```python
from build123d import *

# Parameters (mm, degrees)
F0_R         = 23.8211318964
F0_R_2       = 22.0256608
F3_DEPTH     = 50.17713
F3_FACE_R    = 23.8211318964
F3_FACE_R_2  = 22.0256608
F3_FACE1_R   = 23.8211318964
F3_FACE1_R_2 = 22.0256608
F4_DEPTH     = 2.16738
F1_R         = 2.1104987
F5_DEPTH     = 100.6018
F2_W         = 22.9499428533
F2_H         = 0.7366
F2_W_2       = 0.7306225889
F2_H_2       = 22.9688390891
F2_W_3       = 22.9015578225
F2_H_3       = 22.9767380224
F6_DEPTH     = 36.93024


with BuildPart() as f3:
    # F0 (on Top) → F3 (new body)
    with BuildSketch(Plane.XY):
        Circle(F0_R)
        Circle(F0_R_2, mode=Mode.SUBTRACT)
    extrude(amount=F3_DEPTH)

    # F0 (on Top) + F3_face (on face) + F3_face1 (on face) → F4 (join)
    with BuildSketch(Plane.XY):
        Circle(F0_R)
        Circle(F0_R_2, mode=Mode.SUBTRACT)
        Circle(F0_R_2)
    with BuildSketch(Plane.XY.offset(50.17713)):
        Circle(F3_FACE_R)
        Circle(F3_FACE_R_2, mode=Mode.SUBTRACT)
    with BuildSketch(Plane(origin=(0, 0, 0), x_dir=(1, 0, 0), z_dir=(0, 0, -1))):
        Circle(F3_FACE1_R)
        Circle(F3_FACE1_R_2, mode=Mode.SUBTRACT)
    extrude(amount=F4_DEPTH, dir=(0, 0, 1))

    # F1 (on Top) → F5 (join)
    with BuildSketch(Plane.XY):
        Circle(F1_R)
    extrude(amount=F5_DEPTH)

    # F2 (on Top) → F6 (join)
    with BuildSketch(Plane.XY):
        with Locations((11.8395101745, 0.0209339964)):
            Rectangle(F2_W, F2_H)
        with Locations((-0.0007725466, 0.0209339964)):
            Rectangle(F2_W_2, F2_H)
        with Locations((-0.0007725466, 11.873653541)):
            Rectangle(F2_W_2, F2_H_2)
        with Locations((-11.8168627523, 0.0209339964)):
            Rectangle(F2_W_3, F2_H)
        with Locations((-0.0007725466, -11.8357350148)):
            Rectangle(F2_W_2, F2_H_3)
    extrude(amount=F6_DEPTH)


solid = f3.part
```
Verification items for the finished model (mm, model axes). A direction names the side the tool comes from. Coordinates: 2 decimals unless noted, no trailing zeros. Loops run counter-clockwise (first coordinate to the right, second up) from the corner with the lowest first, then second, coordinate; pieces in that order, holes last. Notation, with made-up numbers: (12.25, -34.75) -> (22.25, -34.75) arc R16 ccw to (22.25, -8.75) -> close; hole circle Ø8 at (64, -37.75). An arc over 180 degrees is marked (long way). Answer in a Markdown table with one row per item.
1) Draft check along X on faces 1 (the face through (0.365, 12, 19)), 2 (the face through (-5.164, -23.255, 25.806)), 3 (the face through (0, 0, 0)). Enter one of: released by +X, released by -X, zero draft, split by the parting line, or undercut.
The answers:
| item | result |
|---|---|
| face 1 | undercut |
| face 2 | split by the parting line |
| face 3 | zero draft |
2) Section check D-D (z = 75.5). Record the cut outline in (x, y).
The answers:
| item | result |
|---|---|
| outline | circle Ø4.22 at (0, 0) |
3) Section check A-A (z = 9.5). Record the cut outline in (x, y), and give its area (3 significant figures).
The answers:
| item | result |
|---|---|
| outline | circle Ø47.64 at (0, 0); hole (-22.02, -0.35) arc R22.03 ccw to (-0.37, -22.02) -> (-0.37, -2.08) arc R2.11 cw to (-2.08, -0.35) -> close; hole (-22.02, 0.39) -> (-2.07, 0.39) arc R2.11 cw to (-0.37, 2.08) -> (-0.37, 22.02) arc R22.03 ccw to start; hole (0.36, -22.02) arc R22.03 ccw to (22.02, -0.35) -> (2.08, -0.35) arc R2.11 cw to (0.36, -2.08) -> close; hole (0.36, 2.08) arc R2.11 cw to (2.07, 0.39) -> (22.02, 0.39) arc R22.03 ccw to (0.36, 22.02) -> close |
| area | 331 mm2 |
4) Section check C-C (y = 19). Record the cut outline in (x, z), and give its area (3 significant figures).
The answers:
| item | result |
|---|---|
| outline | (-14.37, 0) -> (14.37, 0) -> (14.37, 52.34) -> (11.14, 52.34) -> (11.14, 2.17) -> (0.36, 2.17) -> (0.36, 36.93) -> (-0.37, 36.93) -> (-0.37, 2.17) -> (-11.14, 2.17) -> (-11.14, 52.34) -> (-14.37, 52.34) -> close |
| area | 412 mm2 |
5) Access from +Z, -Z, +X, -X, +Y, -Y to the whole of each face (thin tool, end or side, straight path). Record for faces 4 (the face through (0, 0, 100.602)), 5 (the face through (-9, -9, 2.167)).
The answers:
| item | result |
|---|---|
| face 4 | +Z, +X, -X, +Y, -Y |
| face 5 | +Z |
6) Depth check by flat-ended pin: P1, Ø6, axis at x = -7.5, z = 25, coming from the +Y side; P2, Ø12, axis at x = 11.5, z = 50, coming from the +Y side; P3, Ø1, axis at x = 9, z = 29, coming from the -Y side; P4, Ø6, axis at x = -6, z = 64, coming from the +Y side. Enter the tip coordinate at first touch or a pass-through.
The answers:
| item | result |
|---|---|
| P1 | stops at y = 23.39 |
| P2 | stops at y = 23.18 |
| P3 | stops at y = -22.25 |
| P4 | passes through |
7) Scan lines: line 1 along X through (y, z) = (0.5, 36); line 2 along X through (y, z) = (-10.5, 16.5); line 3 along Y through (x, z) = (13, 9.5). Record each from-to range of solid material in increasing order. Write a range as from..to.
The answers:
| item | result |
|---|---|
| line 1 | x = -23.82..-22.02, -2.05..2.05, 22.02..23.82 |
| line 2 | x = -21.38..-19.36, -0.37..0.36, 19.36..21.38 |
| line 3 | y = -19.96..-17.78, -0.35..0.39, 17.78..19.96 |
8) Section check B-B (x = 5). Record the cut outline in (y, z).
The answers:
| item | result |
|---|---|
| outline | (-23.29, 0) -> (23.29, 0) -> (23.29, 52.34) -> (21.45, 52.34) -> (21.45, 2.17) -> (0.39, 2.17) -> (0.39, 36.93) -> (-0.35, 36.93) -> (-0.35, 2.17) -> (-21.45, 2.17) -> (-21.45, 52.34) -> (-23.29, 52.34) -> close |
